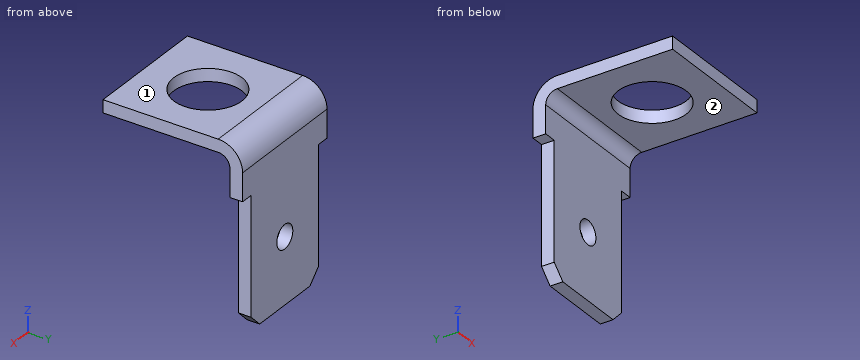
```python
from build123d import *

# Parameters (mm, degrees)
SKETCH_1_W                       = 7.9
SKETCH_1_H                       = 8.8
SM_BASE_FLANGE_1_DEPTH           = 0.8
SM_EDGE_FLANGE_1_STRIP_W         = 4.6732
SM_EDGE_FLANGE_1_STRIP_H         = 0.8
SM_EDGE_FLANGE_1_STRIP_CUT_DEPTH = 7.9
SM_EDGE_FLANGE_1_DEPTH           = 7.9
SKETCH_7_R                       = 2.15
CUT_EXTRUDE_1_DEPTH              = 10
SKETCH_8_W                       = 0.8
SKETCH_8_H                       = 8.2
CUT_EXTRUDE_2_DEPTH              = 10
SKETCH_9_R                       = 0.75
CUT_EXTRUDE_3_DEPTH              = 10
CHAMFER_1_SIZE                   = 0.8


# Sheet-metal steps are written as plain solids
with BuildPart() as part:
    # Sketch 1 → 基体-法兰1 (new body)
    with BuildSketch(Plane.XY):
        Rectangle(SKETCH_1_W, SKETCH_1_H)
    extrude(amount=-SM_BASE_FLANGE_1_DEPTH)

    # 边线-法兰1 strip (across the edge) → 边线-法兰1 strip cut (cut)
    with BuildSketch(Plane(origin=(-3.95, 4.4, -0.8), x_dir=(0, -1, 0), z_dir=(1, 0, 0))):
        with Locations((-0.8, -0.4)):
            Rectangle(SM_EDGE_FLANGE_1_STRIP_W, SM_EDGE_FLANGE_1_STRIP_H)
    extrude(amount=SM_EDGE_FLANGE_1_STRIP_CUT_DEPTH, mode=Mode.SUBTRACT)

    # 边线-法兰1 section (across the edge) → 边线-法兰1 (add)
    with BuildSketch(Plane(origin=(-3.95, 4.4, -0.8), x_dir=(0, -1, 0), z_dir=(1, 0, 0))):
        with BuildLine():
            Line((0, 0.7366), (0, 10.7))
            Line((0, 10.7), (0.8, 10.7))
            Line((0.8, 10.7), (0.8, 0.7366))
            ThreePointArc((0.8, 0.7366), (1.015745145, 0.215745145), (1.5366, 0))
            Line((1.5366, 0), (1.5366, -0.8))
            ThreePointArc((1.5366, -0.8), (0.45005972, -0.34994028), (0, 0.7366))
        make_face()
    extrude(amount=SM_EDGE_FLANGE_1_DEPTH)

    # 草图7 → 切除-拉伸1 (cut)
    with BuildSketch(Plane(origin=(0, 0, -0.8), x_dir=(-1, 0, 0), z_dir=(0, 0, -1))):
        with Locations((0, -0.45)):
            Circle(SKETCH_7_R)
    extrude(amount=-CUT_EXTRUDE_1_DEPTH, mode=Mode.SUBTRACT)

    # 草图8 → 切除-拉伸2 (cut)
    with BuildSketch(Plane(origin=(0, 4.4, 0), x_dir=(1, 0, 0), z_dir=(0, 1, 0))):
        with Locations((3.55, 7.4)):
            Rectangle(SKETCH_8_W, SKETCH_8_H)
        with Locations((-3.55, 7.4)):
            Rectangle(SKETCH_8_W, SKETCH_8_H)
    extrude(amount=-CUT_EXTRUDE_2_DEPTH, mode=Mode.SUBTRACT)

    # 草图9 → 切除-拉伸3 (cut)
    with BuildSketch(Plane(origin=(0, 4.4, 0), x_dir=(1, 0, 0), z_dir=(0, 1, 0))):
        with Locations(Location((0, 7.35, 0), (0, 0, 270))):
            Circle(SKETCH_9_R)
    extrude(amount=-CUT_EXTRUDE_3_DEPTH, mode=Mode.SUBTRACT)

    # 倒角1
    chamfer_1_edges = [part.edges().sort_by_distance(p)[0] for p in [
        (-3.15, 4, -11.5),
        (3.15, 4, -11.5),
    ]]
    chamfer(chamfer_1_edges, length=CHAMFER_1_SIZE)


solid = part.part
```
Work out the finished part from the listing and answer in its coordinate system (mm). Face numbers are marked on the shaded views. A direction names the side the tool comes from. Round coordinates to 2 decimals unless told otherwise and drop trailing zeros. Write each loop counter-clockwise with the first axis right and the second up, starting at its lowest first coordinate (ties: lowest second). Pieces come first, ordered by that corner, then holes. Notation, with made-up numbers: (2, 65.5) - (23, 65.5) arc R24 ccw to (23, 80.5) - close; hole circle Ø4 at (-16.75, 86.25). An arc over 180 degrees is marked (long way). Return JSON: item names as keys, results as strings. Group by question number.
Q1. The part is cut by section B-B on y = -0.45. Write down the section's boundary in (x, z), then the cut area to 3 significant figures.
Q2. The part is cut by section D-D on x = 2.5. Write down the section's boundary in (y, z).
Q3. For the marked faces 1 and 2, determine the directions among +Z, -Z, +X, -X, +Y, -Y from which every point of the face is accessible in a straight line to the end or side of a thin tool.
Q4. Each of these flat-tipped pins is pushed along its axis until it touches: pin 1 Ø1.7 at (x, z) = (0, -7.35) entering from +Y; pin 2 Ø3 at (x, z) = (3, -4) entering from -Y; pin 3 Ø0.6 at (x, y) = (-3.5, 4) entering from -Z; pin 4 Ø0.9 at (y, z) = (4, -8.5) entering from -X. Where does it stop, or does it pass through?
Q5. Find the intervals of material crossed by L1, parallel to X at y = 3.8, z = -7.35; L2, parallel to Z at x = 0, y = -3.5; L3, parallel to Y at x = -0.5, z = -8.25, in increasing order.
Q6. The part is cut by section A-A on x = 0. Write down the section's boundary in (y, z).
Q7. The part is cut by section C-C on z = -7.35. Write down the section's boundary in (x, y).
Solved:
{
 "1": {"outline": "(-3.95, -0.8) - (-2.15, -0.8) - (-2.15, 0) - (-3.95, 0) - close; (2.15, -0.8) - (3.95, -0.8) - (3.95, 0) - (2.15, 0) - close", "area": "2.88 mm²"},
 "2": {"outline": "(-4.4, -0.8) - (2.86, -0.8) arc R0.74 cw to (3.6, -1.54) - (3.6, -11.35) - (4.4, -11.35) - (4.4, -1.54) arc R1.54 ccw to (2.86, 0) - (-4.4, 0) - close"},
 "3": {"face 1": "+Z, +X, -X, +Y, -Y", "face 2": "-Z, +X, -X, -Y"},
 "4": {"pin 1": "y = 4.4", "pin 2": "y = 3.6", "pin 3": "z = -3.3", "pin 4": "x = -3.15"},
 "5": {"L1": "-3.15 to -0.75, 0.75 to 3.15", "L2": "-0.8 to 0", "L3": "3.6 to 4.4"},
 "6": {"outline": "(-4.4, -0.8) - (-2.6, -0.8) - (-2.6, 0) - (-4.4, 0) - close; (1.7, -0.8) - (2.86, -0.8) arc R0.74 cw to (3.6, -1.54) - (3.6, -6.6) - (4.4, -6.6) - (4.4, -1.54) arc R1.54 ccw to (2.86, 0) - (1.7, 0) - close; (3.6, -11.5) - (4.4, -11.5) - (4.4, -8.1) - (3.6, -8.1) - close"},
 "7": {"outline": "(-3.15, 3.6) - (-0.75, 3.6) - (-0.75, 4.4) - (-3.15, 4.4) - close; (0.75, 3.6) - (3.15, 3.6) - (3.15, 4.4) - (0.75, 4.4) - close"}
}
